```python
from build123d import *

# Parameters (mm, degrees)
F0_W      = 76.2
F0_H      = 76.2
F1_DEPTH  = 76.2
F2_W      = 25.4
F2_H      = 25.4
F3_DEPTH  = 12.7
F4_R      = 12.7
F5_DEPTH  = 12.7
F7_D      = 25.4
F8_W      = 49.319143
F8_H      = 46.700371
F9_DEPTH  = 12.7
F10_W     = 29.316643
F10_H     = 28.858568
F11_DEPTH = 12.7


with BuildPart() as f1:
    # F0 (on Front) → F1 (new body)
    with BuildSketch(Plane.XZ):
        with Locations((3.721774, 0.220706)):
            Rectangle(F0_W, F0_H)
    extrude(amount=F1_DEPTH)

    # F2 (on face) → F3 (join)
    with BuildSketch(Plane.XZ.offset(76.2)):
        with Locations((3.721774, 0.220706)):
            Rectangle(F2_W, F2_H)
    extrude(amount=F3_DEPTH)

    # F4 (on face) → F5 (join)
    with BuildSketch(Plane.YZ.offset(41.821774)):
        with Locations((-38.1, 0.220706)):
            Circle(F4_R)
    extrude(amount=F5_DEPTH)

    # F7 (through all)
    with Locations(Plane.XY.offset(38.320706)):
        with Locations((3.721774, -38.1)):
            Hole(F7_D / 2)

    # F8 (on face) → F9 (join)
    with BuildSketch(Plane(origin=(-34.378226, 0, 0), x_dir=(0, -1, 0), z_dir=(-1, 0, 0))):
        with Locations((37.359572, -1.829109)):
            Rectangle(F8_W, F8_H)
    extrude(amount=F9_DEPTH)

    # F10 (on face) → F11 (join)
    with BuildSketch(Plane(origin=(-47.078226, 0, 0), x_dir=(0, -1, 0), z_dir=(-1, 0, 0))):
        with Locations((37.96064, -3.749257)):
            Rectangle(F10_W, F10_H)
    extrude(amount=F11_DEPTH)


solid = f1.part
```
Geometry: final body of the model. Coordinates: model frame, mm. A direction names the side the tool comes from. Give positions to 0.01 mm unless a question says otherwise; leave off trailing zeros. Write each loop counter-clockwise with the first axis right and the second up, starting at its lowest first coordinate (ties: lowest second). Pieces come first, ordered by that corner, then holes.
1. Section query D-D, the plane y = -17.5. Return loops of the section in (x, z).
2. Reachability of faces 4 (the flat face through (-53, -52.619, -4)), 5 (the flat face through (-41, -12.7, -2)), 6 (the flat face through (41.822, -29, -9)) from +Z, -Z, +X, -X, +Y, -Y: full face, straight path, thin tool, end or side. Return the list, or none.
3. Section query B-B, the plane x = 3.5. Return loops of the section in (y, z), then the cut area to 3 significant figures.
4. Pin query (flat end, axial travel): P1, Ø14, axis at y = -82, z = -5, coming from the +X side; P2, Ø6.5, axis at x = -40.5, z = -13.5, coming from the +Y side; P3, Ø4, axis at x = 5, y = -82, coming from the +Z side; P4, Ø20.5, axis at x = 3.72, y = -38.1, coming from the -Z side. Return the tip coordinate at first contact, or that it passes through.
5. Line query: probe 1 along X at (y, z) = (-38, 14); probe 2 along X at (y, z) = (-69, 18); probe 3 along Y at (x, z) = (-48, 3). Output: solid intervals per line, ascending.
6. Draft query along X for faces 1 (the flat face through (-8.978, -82, 0)), 2 (the cylindrical face through (6.47, -50.5, -0.31)), 3 (the flat face through (-14, -38, -37.879)). Return one class per face: released by +X, released by -X, zero draft, split by the parting line, or undercut.
7. Section query C-C, the plane z = 2.5. Return loops of the section in (x, y).
8. Section query A-A, the plane y = -38.1. Return loops of the section in (x, z).
Computed:
1. outline: (-47.08, -25.18) - (-34.38, -25.18) - (-34.38, -37.88) - (41.82, -37.88) - (41.82, 38.32) - (-34.38, 38.32) - (-34.38, 21.52) - (-47.08, 21.52) - close
2. face 4: +Z, -Z, -X, -Y
2. face 5: +Z, -Z, -X, +Y
2. face 6: +X
3. outline: (-88.9, -12.48) - (-76.2, -12.48) - (-76.2, -37.88) - (-50.8, -37.88) - (-50.8, 38.32) - (-76.2, 38.32) - (-76.2, 12.92) - (-88.9, 12.92) - close; (-25.4, -37.88) - (0, -37.88) - (0, 38.32) - (-25.4, 38.32) - close
3. area: 4,190 mm2
4. P1: stops at x = 41.82
4. P2: stops at y = -12.7
4. P3: stops at z = 12.92
4. P4: passes through
5. probe 1: x = -47.08 to -8.98, 16.42 to 41.82
5. probe 2: x = -34.38 to 41.82
5. probe 3: y = -52.62 to -23.3
6. face 1: released by -X
6. face 2: undercut
6. face 3: zero draft
7. outline: (-59.78, -52.62) - (-47.08, -52.62) - (-47.08, -62.02) - (-34.38, -62.02) - (-34.38, -76.2) - (-8.98, -76.2) - (-8.98, -88.9) - (16.42, -88.9) - (16.42, -76.2) - (41.82, -76.2) - (41.82, -50.59) - (54.52, -50.59) - (54.52, -25.61) - (41.82, -25.61) - (41.82, 0) - (-34.38, 0) - (-34.38, -12.7) - (-47.08, -12.7) - (-47.08, -23.3) - (-59.78, -23.3) - close; hole circle Ø25.4 at (3.72, -38.1)
8. outline: (-59.78, -18.18) - (-47.08, -18.18) - (-47.08, -25.18) - (-34.38, -25.18) - (-34.38, -37.88) - (-8.98, -37.88) - (-8.98, 38.32) - (-34.38, 38.32) - (-34.38, 21.52) - (-47.08, 21.52) - (-47.08, 10.68) - (-59.78, 10.68) - close; (16.42, -37.88) - (41.82, -37.88) - (41.82, -12.48) - (54.52, -12.48) - (54.52, 12.92) - (41.82, 12.92) - (41.82, 38.32) - (16.42, 38.32) - close
